Here's how the part is built. I have some questions about the finished solid (model axes, mm). A direction names the side the tool comes from. Coordinates: 2 decimals unless noted, no trailing zeros. Write each loop counter-clockwise with the first axis right and the second up, starting at its lowest first coordinate (ties: lowest second). Pieces come first, ordered by that corner, then holes.
(1) Imagine slicing it at C-C, the plane x = 25. List the corners of the cut face in (y, z) for me.
(2) For pin 1 Ø10 at (x, z) = (5, -33) entering from +Y; pin 2 Ø4 at (y, z) = (-2.5, -14.5) entering from -X; pin 3 Ø1.5 at (x, y) = (-3, 5.5) entering from +Z; pin 4 Ø1.5 at (x, z) = (15.5, -4.5) entering from -Y, each with a flat end and sliding along its axis, tell me the tip position at first contact or that it passes through.
(3) Please list where these lines run through material, in increasing order: probe 1 along X at (y, z) = (-0.25, 6.5); probe 2 along Y at (x, z) = (12.5, -61); probe 3 along Z at (x, y) = (9, 1.25).
(4) Imagine slicing it at B-B, the plane y = 9.5. List the corners of the cut face in (x, z) for me, plus the area to 3 significant figures.
(5) Imagine slicing it at A-A, the plane z = 5. List the corners of the cut face in (x, y) for me.
(6) Imagine slicing it at D-D, the plane y = 4. List the corners of the cut face in (x, z) for me, plus the area to 3 significant figures.
(7) Which directions (+Z, -Z, +X, -X, +Y, -Y) give clear straight access to the entire face, cutting with the end or side of a thin tool? Please do faces 4 (the flat face through (17.5, -2, 0)), 5 (the flat face through (-3, 0, 5)), 6 (the flat face through (17.5, 9, 0)), 7 (the flat face through (0, 3, -41)).
(8) Thinking about a two-plate mould opening in Y: for faces 1 (the flat face through (10, 3, 0)), 2 (the flat face through (-3, -5, 0)), 3 (the flat face through (2.5, -2, 0)), which applies, released by +Y, released by -Y, zero draft, split by the parting line, or undercut?
```python
from build123d import *

# Parameters (mm, degrees)
SKETCH1_W           = 20
SKETCH1_H           = 73.625466435
BOSS_EXTRUDE1_DEPTH = 7
SKETCH2_W           = 10
SKETCH2_H           = 10
BOSS_EXTRUDE2_DEPTH = 5
SKETCH3_W           = 10
SKETCH3_H           = 5
BOSS_EXTRUDE3_DEPTH = 10
SKETCH4_W           = 7.5
SKETCH4_H           = 10
BOSS_EXTRUDE4_DEPTH = 3.5


with BuildPart() as part:
    # Sketch1 → Boss-Extrude1 (new body)
    with BuildSketch(Plane(origin=(0, 0, 0), x_dir=(1, 0, 0), z_dir=(0, 1, 0))):
        with Locations((10, 36.812733218)):
            Rectangle(SKETCH1_W, SKETCH1_H)
    extrude(amount=BOSS_EXTRUDE1_DEPTH)

    # Sketch2 → Boss-Extrude2 (add)
    with BuildSketch(Plane(origin=(0, 7, 0), x_dir=(1, 0, 0), z_dir=(0, 1, 0))):
        with Locations((-2.5, 5)):
            Rectangle(SKETCH2_W, SKETCH2_H)
        with Locations((22.5, 5)):
            Rectangle(SKETCH2_W, SKETCH2_H)
    boss_extrude2 = extrude(amount=BOSS_EXTRUDE2_DEPTH)

    # Sketch3 → Boss-Extrude3 (add)
    with BuildSketch(Plane.XY):
        with Locations((-2.5, 9.5)):
            Rectangle(SKETCH3_W, SKETCH3_H)
        with Locations((22.5, 9.5)):
            Rectangle(SKETCH3_W, SKETCH3_H)
    boss_extrude3 = extrude(amount=BOSS_EXTRUDE3_DEPTH)

    # Sketch4 → Boss-Extrude4 (add)
    with BuildSketch(Plane.XZ.offset(-7)):
        with Locations((-3.75, -5)):
            Rectangle(SKETCH4_W, SKETCH4_H)
        with Locations((23.75, -5)):
            Rectangle(SKETCH4_W, SKETCH4_H)
    boss_extrude4 = extrude(amount=BOSS_EXTRUDE4_DEPTH)

    # Mirror1: Boss-Extrude2, Boss-Extrude3, Boss-Extrude4 across plane
    add(boss_extrude2.mirror(Plane.ZX.offset(3.5)))
    add(boss_extrude3.mirror(Plane.ZX.offset(3.5)))
    add(boss_extrude4.mirror(Plane.ZX.offset(3.5)))


solid = part.part
```
Recorded:
1. outline: (-5, -10) - (12, -10) - (12, 10) - (7, 10) - (7, 0) - (0, 0) - (0, 10) - (-5, 10) - close
2. pin 1: stops at y = 7
2. pin 2: passes through
2. pin 3: stops at z = 0
2. pin 4: stops at y = 0
3. probe 1: x = -7.5 to 2.5, 17.5 to 27.5
3. probe 2: y = 0 to 7
3. probe 3: z = -73.63 to 0
4. outline: (-7.5, -10) - (2.5, -10) - (2.5, 10) - (-7.5, 10) - close; (17.5, -10) - (27.5, -10) - (27.5, 10) - (17.5, 10) - close
4. area: 400 mm2
5. outline: (-7.5, -5) - (2.5, -5) - (2.5, 0) - (-7.5, 0) - close; (-7.5, 7) - (2.5, 7) - (2.5, 12) - (-7.5, 12) - close; (17.5, -5) - (27.5, -5) - (27.5, 0) - (17.5, 0) - close; (17.5, 7) - (27.5, 7) - (27.5, 12) - (17.5, 12) - close
6. outline: (-7.5, -10) - (0, -10) - (0, -73.63) - (20, -73.63) - (20, -10) - (27.5, -10) - (27.5, 0) - (-7.5, 0) - close
6. area: 1,620 mm2
7. face 4: +Z, -Z, -Y
7. face 5: +Z, +X, -X
7. face 6: +Z, -Z, +Y
7. face 7: -Z, -X, +Y, -Y
8. face 1: undercut
8. face 2: released by -Y
8. face 3: zero draft
